Model file for the job. Use its own axes, mm. Face numbers are marked on the shaded views. Coordinates: 2 decimals unless noted, no trailing zeros. Write each loop counter-clockwise with the first axis right and the second up, starting at its lowest first coordinate (ties: lowest second). Pieces come first, ordered by that corner, then holes. Notation, with made-up numbers: (-30, 11.25) - (-2, 11.25) arc R25 cw to (-2, 25.25) - close; hole circle Ø6 at (68.5, 47). An arc over 180 degrees is marked (long way). Put each result on its own line as item: value. Start each with the question number.
1. Saw through at D-D, the plane y = 0. Write the cut outline in (x, z).
2. Saw through at A-A, the plane y = -8. Write the cut outline in (x, z).
3. Saw through at C-C, the plane z = -1.3. Write the cut outline in (x, y), plus the area to 3 significant figures.
4. Pull direction Z, two halves, no side cores. Call the marked faces 1, 2 and 3: released by +Z, released by -Z, zero draft, split by the parting line, or undercut.
5. Saw through at B-B, the plane z = 0.95. Write the cut outline in (x, y).
6. Drop flat-ended pins along their axis: P1, Ø7, axis at x = 5.5, y = 4, coming from the +Z side; P2, Ø1.5, axis at x = -2, z = -1, coming from the +Y side. Give the stop position or say it passes through.
7. Drill centre lines: L1, parallel to X at y = -1, z = 0.6; L2, parallel to X at y = 4, z = 1.15; L3, parallel to Z at x = 2.5, y = 1.5. Where is each one in solid material? Low to high. Write a range as from..to.
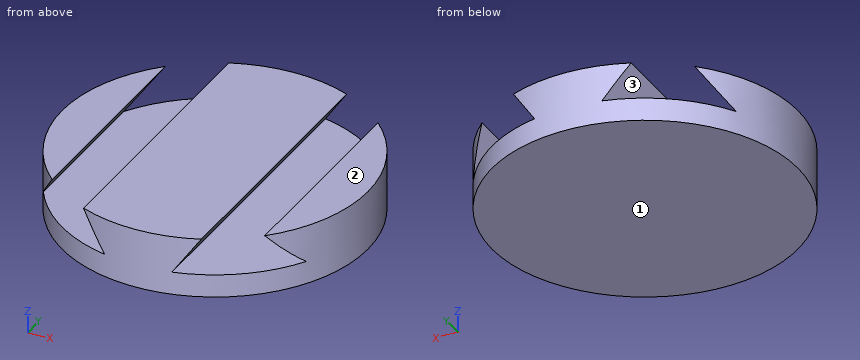
```python
from build123d import *

# Parameters (mm, degrees)
F0_R     = 10
F1_DEPTH = 3.9
F4_DEPTH = 25
F5_DEPTH = 25


with BuildPart() as f1:
    # F0 (on Top) → F1 (new body)
    with BuildSketch(Plane.XY):
        Circle(F0_R)
    extrude(amount=F1_DEPTH)


with BuildPart() as f1_1:
    # F3: moved
    add(f1.part.moved(Location((0, 0, -2.5))))

    # F2 (on Front) → F4 (cut)
    with BuildSketch(Plane.XZ):
        Polygon((-2.2, -1), (-3.849474, 1.4), (-6.950526, 1.4), (-8.6, -1), align=None)
        Polygon((8.6, -1), (6.950526, 1.4), (3.849474, 1.4), (2.2, -1), align=None)
    extrude(amount=-F4_DEPTH, mode=Mode.SUBTRACT)

    # F4_face (on face) → F5 (cut)
    with BuildSketch(Plane(origin=(5.4, 0, 0.061112), x_dir=(1, 0, 0), z_dir=(0, 1, 0))):
        Polygon((1.550526, -1.338888), (3.2, 1.061112), (-3.2, 1.061112), (-1.550526, -1.338888), align=None)
        Polygon((-14, 1.061112), (-12.350526, -1.338888), (-9.249474, -1.338888), (-7.6, 1.061112), align=None)
    extrude(amount=-F5_DEPTH, mode=Mode.SUBTRACT)


solid = f1_1.part
```
Final values:
1. outline: (-10, -2.5) - (10, -2.5) - (10, 1.4) - (6.95, 1.4) - (8.6, -1) - (2.2, -1) - (3.85, 1.4) - (-3.85, 1.4) - (-2.2, -1) - (-8.6, -1) - (-6.95, 1.4) - (-10, 1.4) - close
2. outline: (-6, -2.5) - (6, -2.5) - (6, -1) - (2.2, -1) - (3.85, 1.4) - (-3.85, 1.4) - (-2.2, -1) - (-6, -1) - close
3. outline: circle Ø20 at (0, 0)
3. area: 314 mm²
4. face 1: released by -Z
4. face 2: released by +Z
4. face 3: undercut
5. outline: (-7.26, -6.88) - (-7.26, 6.88) arc R10 ccw to start; (-3.54, -9.35) arc R10 ccw to (3.54, -9.35) - (3.54, 9.35) arc R10 ccw to (-3.54, 9.35) - close; (7.26, -6.88) arc R10 ccw to (7.26, 6.88) - close
6. P1: stops at z = 1.4
6. P2: stops at y = 9.92
7. L1: x = -9.95..-7.5, -3.3..3.3, 7.5..9.95
7. L2: x = -9.17..-7.12, -3.68..3.68, 7.12..9.17
7. L3: z = -2.5..-1, -0.56..1.4
